Here's how the part is built. I have some questions about the finished solid (model axes, mm). Face numbers are marked on the shaded views. A direction names the side the tool comes from. Round coordinates to 2 decimals unless told otherwise and drop trailing zeros. Order: outer loops, then holes, each group sorted by start corner. A loop starts at its lowest first (then second) coordinate and runs counter-clockwise, first axis right, second up. Notation, with made-up numbers: M 17.5,35 L 31.5,35 A10 ccw 31.5,48 Z; hole C 1,55.5 d10. An arc over 180 degrees is marked long. Write item = value, one per line. Start each with the question number.
Item 1: I want a section at A-A, the plane x = -22.5. List the corners of the cut face in (y, z) for me.
Item 2: I want a section at B-B, the plane z = 37.5. List the corners of the cut face in (x, y) for me, plus the area to 3 significant figures.
Item 3: I want a section at C-C, the plane y = -5.5. List the corners of the cut face in (x, z) for me.
Item 4: For the marked faces 4, 5, 6 and 7, which set-ups out of +Z, -Z, +X, -X, +Y, -Y let a thin tool reach every point of the face, with its end or its side?
Item 5: We'd pull the mould along X, two halves only. Please class the marked faces 1, 2 and 3: pulls with the +X half, pulls with the -X half, needs draft (parallel to the pull), parting line crosses it, or undercut.
Item 6: I'm going to push flat-ended pins straight in: P1, Ø10.5, axis at y = -5.5, z = 15, coming from the -X side; P2, Ø4, axis at x = 11, z = -7, coming from the -Y side; P3, Ø7, axis at y = -24.5, z = 15, coming from the -X side; P4, Ø5, axis at x = 12, z = 27.5, coming from the -Y side. Where does each tip first touch, or does it pass through?
Item 7: Please list where these lines run through material, in increasing order: L1, parallel to X at y = 31.6, z = -7.5; L2, parallel to Y at x = 24.75, z = 15; L3, parallel to Y at x = 25.5, z = 18.5.
Item 8: I want a section at D-D, the plane y = -18.5. List the corners of the cut face in (x, z) for me.
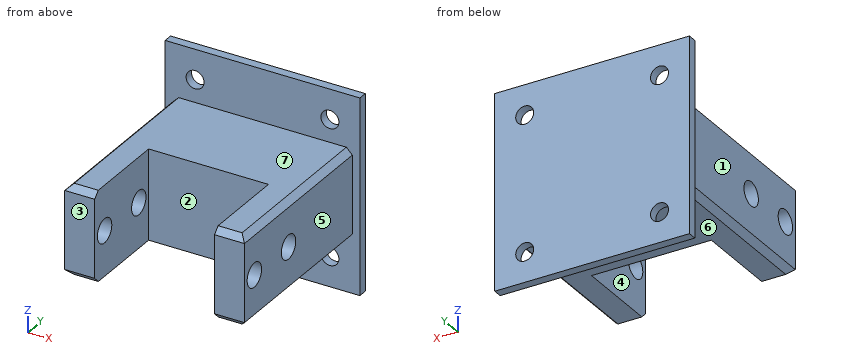
```python
from build123d import *

# Parameters (mm, degrees)
EXTRUDE_1_DEPTH     = 30
SKETCH_2_R          = 4
CUT_EXTRUDE_1_DEPTH = 74.484692283
SKETCH_3_W          = 65
SKETCH_3_H          = 65
SKETCH_3_R          = 3
EXTRUDE_2_DEPTH     = 3
CHAMFER_2_SIZE      = 2


with BuildPart() as part:
    # 草图1 → 凸台-拉伸1 (new body)
    with BuildSketch(Plane.XY):
        Polygon((-30, -30), (-20, -30), (-20, 0), (20, 0), (20, -30), (30, -30), (30, 30), (-30, 30), align=None)
    extrude(amount=EXTRUDE_1_DEPTH)

    # 草图2 → 切除-拉伸1 (cut, through all)
    with BuildSketch(Plane.ZY.offset(30)):
        with Locations((15, -5.5)):
            Circle(SKETCH_2_R)
        with Locations((15, -24.5)):
            Circle(SKETCH_2_R)
    extrude(amount=-CUT_EXTRUDE_1_DEPTH, mode=Mode.SUBTRACT)

    # 草图3 → 凸台-拉伸2 (add)
    with BuildSketch(Plane(origin=(0, 30, 0), x_dir=(1, 0, 0), z_dir=(0, 1, 0))):
        with Locations((0, -15)):
            Rectangle(SKETCH_3_W, SKETCH_3_H)
        with Locations(Location((22.5, -37.5, 0), (0, 0, 270))):
            Circle(SKETCH_3_R, mode=Mode.SUBTRACT)
        with Locations(Location((-22.5, -37.5, 0), (0, 0, 270))):
            Circle(SKETCH_3_R, mode=Mode.SUBTRACT)
        with Locations(Location((-22.5, 7.5, 0), (0, 0, 270))):
            Circle(SKETCH_3_R, mode=Mode.SUBTRACT)
        with Locations(Location((22.5, 7.5, 0), (0, 0, 270))):
            Circle(SKETCH_3_R, mode=Mode.SUBTRACT)
    extrude(amount=EXTRUDE_2_DEPTH)

    # 倒角2
    chamfer_2_edges = [part.edges().sort_by_distance(p)[0] for p in [
        (-25, -30, 0),
        (-30, 0, 0),
        (25, -30, 30),
        (30, 0, 30),
        (-30, 0, 30),
        (-25, -30, 30),
        (30, 0, 0),
        (25, -30, 0),
    ]]
    chamfer(chamfer_2_edges, length=CHAMFER_2_SIZE)


solid = part.part
```
Filled in:
q1.outline = M -30,2 L -28,0 L 30,0 L 30,-4.5 L 33,-4.5 L 33,34.5 L 30,34.5 L 30,30 L -28,30 L -30,28 Z; M 30,-17.5 L 33,-17.5 L 33,-10.5 L 30,-10.5 Z; M 30,40.5 L 33,40.5 L 33,47.5 L 30,47.5 Z; hole C -24.5,15 d8; hole C -5.5,15 d8
q2.outline = M -32.5,30 L -25.5,30 L -25.5,33 L -32.5,33 Z; M -19.5,30 L 19.5,30 L 19.5,33 L -19.5,33 Z; M 25.5,30 L 32.5,30 L 32.5,33 L 25.5,33 Z
q2.area = 159 mm^2
q3.outline = M -30,2 L -28,0 L -20,0 L -20,11 L -30,11 Z; M -30,19 L -20,19 L -20,30 L -28,30 L -30,28 Z; M 20,0 L 28,0 L 30,2 L 30,11 L 20,11 Z; M 20,19 L 30,19 L 30,28 L 28,30 L 20,30 Z
q4.face_4 = +Z, -Z, -Y
q4.face_5 = +Z, -Z, +X, -Y
q4.face_6 = -Z, +X, -X, -Y
q4.face_7 = +Z, +X, -X, -Y
q5.face_1 = pulls with the -X half
q5.face_2 = undercut
q5.face_3 = needs draft
q6.P1 = -30
q6.P2 = 30
q6.P3 = through
q6.P4 = 0
q7.L1 = -32.5 to -25.5, -19.5 to 19.5, 25.5 to 32.5
q7.L2 = -30 to -28.5, -20.5 to -9.5, -1.5 to 33
q7.L3 = -30 to -26.44, -22.56 to -7.44, -3.56 to 33
q8.outline = M -30,2 L -28,0 L -20,0 L -20,30 L -28,30 L -30,28 Z; M 20,0 L 28,0 L 30,2 L 30,28 L 28,30 L 20,30 Z
